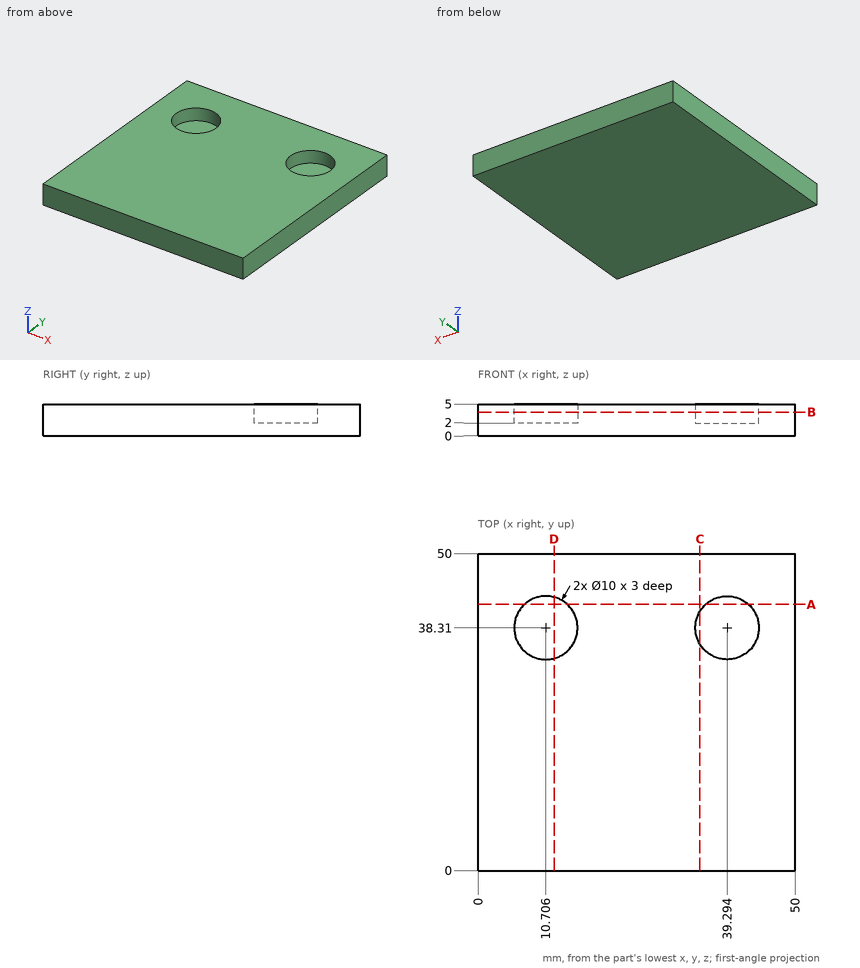
The figure shows three views and two pictorial views of one solid part (mm, origin at its lowest corner). Answer the questions. Round coordinates to 2 decimals unless told otherwise and drop trailing zeros. Order: outer loops, then holes, each group sorted by start corner. A loop starts at its lowest first (then second) coordinate and runs counter-clockwise, first axis right, second up. Notation, with made-up numbers: (52.25, 41.25) - (109.25, 41.25) arc R26 ccw to (109.25, 76.25) - close; hole circle Ø6 at (83, 78). An arc over 180 degrees is marked (long way). Write item = value, one per line. Start each with the question number.
1) Section A-A, the plane y = 42 is taken. Write down the section's boundary in (x, z), plus the area to 4 significant figures.
2) Section C-C, the plane x = 35 is taken. Write down the section's boundary in (y, z), plus the area to 3 significant figures.
3) Given pin 1 (5 mm diameter, centred on x = 9.5, y = 39, fed in from +Z); pin 2 (1 mm diameter, centred on x = 19, z = 2.5, fed in from -Y), each flat-ended and moving along its own axis, determine where each tip first touches the part or whether it passes through.
4) Section B-B, the plane z = 3.7 is taken. Write down the section's boundary in (x, y).
5) Straight lines are drawn through the part: L1, parallel to Y at x = 39, z = 4.65; L2, parallel to X at y = 35.5, z = 3.4; L3, parallel to X at y = 40, z = 2.5. For each, find the intervals that lie inside material, in ascending order.
6) Section D-D, the plane x = 12 is taken. Write down the section's boundary in (y, z), plus the area to 3 significant figures.
Results list:
q1.outline = (0, 0) - (50, 0) - (50, 5) - (42.67, 5) - (42.67, 2) - (35.92, 2) - (35.92, 5) - (14.08, 5) - (14.08, 2) - (7.33, 2) - (7.33, 5) - (0, 5) - close
q1.area = 209.5 mm^2
q2.outline = (0, 0) - (50, 0) - (50, 5) - (40.87, 5) - (40.87, 2) - (35.75, 2) - (35.75, 5) - (0, 5) - close
q2.area = 235 mm^2
q3.pin_1 = 2
q3.pin_2 = 0
q4.outline = (0, 0) - (50, 0) - (50, 50) - (0, 50) - close; hole circle Ø10 at (10.71, 38.31); hole circle Ø10 at (39.29, 38.31)
q5.L1 = 0 to 33.32, 43.3 to 50
q5.L2 = 0 to 6.57, 14.84 to 35.16, 43.43 to 50
q5.L3 = 0 to 6, 15.41 to 34.59, 44 to 50
q6.outline = (0, 0) - (50, 0) - (50, 5) - (43.14, 5) - (43.14, 2) - (33.48, 2) - (33.48, 5) - (0, 5) - close
q6.area = 221 mm^2
